Read the model definition and answer for the solid it produces. Units are mm, in the model's axes. A direction names the side the tool comes from. Coordinates: 2 decimals unless noted, no trailing zeros. Write each loop counter-clockwise with the first axis right and the second up, starting at its lowest first coordinate (ties: lowest second). Pieces come first, ordered by that corner, then holes. Notation, with made-up numbers: (65, 29) -> (100, 29) arc R34 cw to (100, 59) -> close; hole circle Ø7 at (68.5, -33). An arc over 180 degrees is marked (long way). Answer in a Markdown table with one row per item. Add a question column.
Item 1: Straight lines are drawn through the part: line 1 (Y direction, x = -5, z = 1.6); line 2 (X direction, y = 7, z = 1.9); line 3 (Y direction, x = 5.5, z = 1.35). For each, find the intervals that lie inside material, in ascending order. Write a range as from..to.
Item 2: For a pull along Y with two mould halves and no side action, classify faces 1 (the face through (8.25, 0, 1)), 2 (the face through (-5, -5, 2)), 3 (the face through (0, -14, 1)) as +Y half, -Y half, draft (parallel to the pull), parting line (faces both ways), or undercut.
Item 3: Section B-B on z = 2.6 is taken. Write down the section's boundary in (x, y) (3 decimals), then the cut area to 3 significant figures.
Item 4: Section C-C on y = -7 is taken. Write down the section's boundary in (x, z), then the cut area to 3 significant figures.
Item 5: Which of the six approach directions +Z, -Z, +X, -X, +Y, -Y give full straight-line access (tool end or side, diameter ignored) to faces 4 (the face through (0, -1, 0)), 5 (the face through (4.125, -12, 2)), 6 (the face through (-8.25, 0, 1)), 7 (the face through (-3.25, 6, 2)), 8 (the face through (-6, -11, 1))?
Item 6: Section A-A on x = -3.75 is taken. Write down the section's boundary in (y, z).
Item 7: Given pin 1 Ø0.9 at (x, z) = (-5.5, 1) entering from -Y; pin 2 Ø8 at (x, y) = (-4.5, -4.5) entering from -Z, each flat-ended and moving along its own axis, determine where each tip first touches the part or whether it passes through.
Item 8: Section D-D on x = 5.25 is taken. Write down the section's boundary in (y, z), then the cut area to 3 significant figures.
```python
from build123d import *

# Parameters (mm, degrees)
SKETCH1_W           = 16.5
SKETCH1_H           = 22
BOSS_EXTRUDE1_DEPTH = 3
SKETCH2_W           = 8.25
SKETCH2_H           = 3
BOSS_EXTRUDE2_DEPTH = 3
SKETCH3_W           = 3
SKETCH3_H           = 3
CUT_EXTRUDE1_DEPTH  = 3


with BuildPart() as part:
    # Sketch1 → Boss-Extrude1 (new body)
    with BuildSketch(Plane.XY):
        Rectangle(SKETCH1_W, SKETCH1_H)
    extrude(amount=BOSS_EXTRUDE1_DEPTH)

    # Sketch2 → Boss-Extrude2 (add)
    with BuildSketch(Plane(origin=(0, -11, 0), x_dir=(-1, 0, 0), z_dir=(0, -1, 0))):
        with Locations((0, -1.5)):
            Rectangle(SKETCH2_W, SKETCH2_H)
    extrude(amount=BOSS_EXTRUDE2_DEPTH)

    # Sketch3 → Cut-Extrude1 (cut)
    with BuildSketch(Plane.XY.offset(3)):
        with Locations((-4.75, -6.5)):
            Rectangle(SKETCH3_W, SKETCH3_H)
        with Locations((-4.75, 6.5)):
            Rectangle(SKETCH3_W, SKETCH3_H)
    extrude(amount=-CUT_EXTRUDE1_DEPTH, mode=Mode.SUBTRACT)


solid = part.part
```
Results below:
| question | item | result |
|---|---|---|
| 1 | line 1 | y = -11..-8, -5..5, 8..11 |
| 1 | line 2 | x = -8.25..-6.25, -3.25..8.25 |
| 1 | line 3 | y = -11..11 |
| 2 | face 1 | draft |
| 2 | face 2 | undercut |
| 2 | face 3 | -Y half |
| 3 | outline | (-8.25, -11) -> (-4.125, -11) -> (-4.125, -14) -> (4.125, -14) -> (4.125, -11) -> (8.25, -11) -> (8.25, 11) -> (-8.25, 11) -> close; hole (-6.25, -8) -> (-3.25, -8) -> (-3.25, -5) -> (-6.25, -5) -> close; hole (-6.25, 5) -> (-3.25, 5) -> (-3.25, 8) -> (-6.25, 8) -> close |
| 3 | area | 370 mm2 |
| 4 | outline | (-8.25, 0) -> (-6.25, 0) -> (-6.25, 3) -> (-8.25, 3) -> close; (-3.25, 0) -> (8.25, 0) -> (8.25, 3) -> (-3.25, 3) -> close |
| 4 | area | 40.5 mm2 |
| 5 | face 4 | -Z, +X, -X, +Y, -Y |
| 5 | face 5 | +Z, -Z, +X, -Y |
| 5 | face 6 | +Z, -Z, -X, +Y, -Y |
| 5 | face 7 | +Z, -Z |
| 5 | face 8 | +Z, -Z, -X, -Y |
| 6 | outline | (-14, 0) -> (-8, 0) -> (-8, 3) -> (-14, 3) -> close; (-5, 0) -> (5, 0) -> (5, 3) -> (-5, 3) -> close; (8, 0) -> (11, 0) -> (11, 3) -> (8, 3) -> close |
| 7 | pin 1 | stops at y = -11 |
| 7 | pin 2 | stops at z = 0 |
| 8 | outline | (-11, 0) -> (11, 0) -> (11, 3) -> (-11, 3) -> close |
| 8 | area | 66.0 mm2 |
